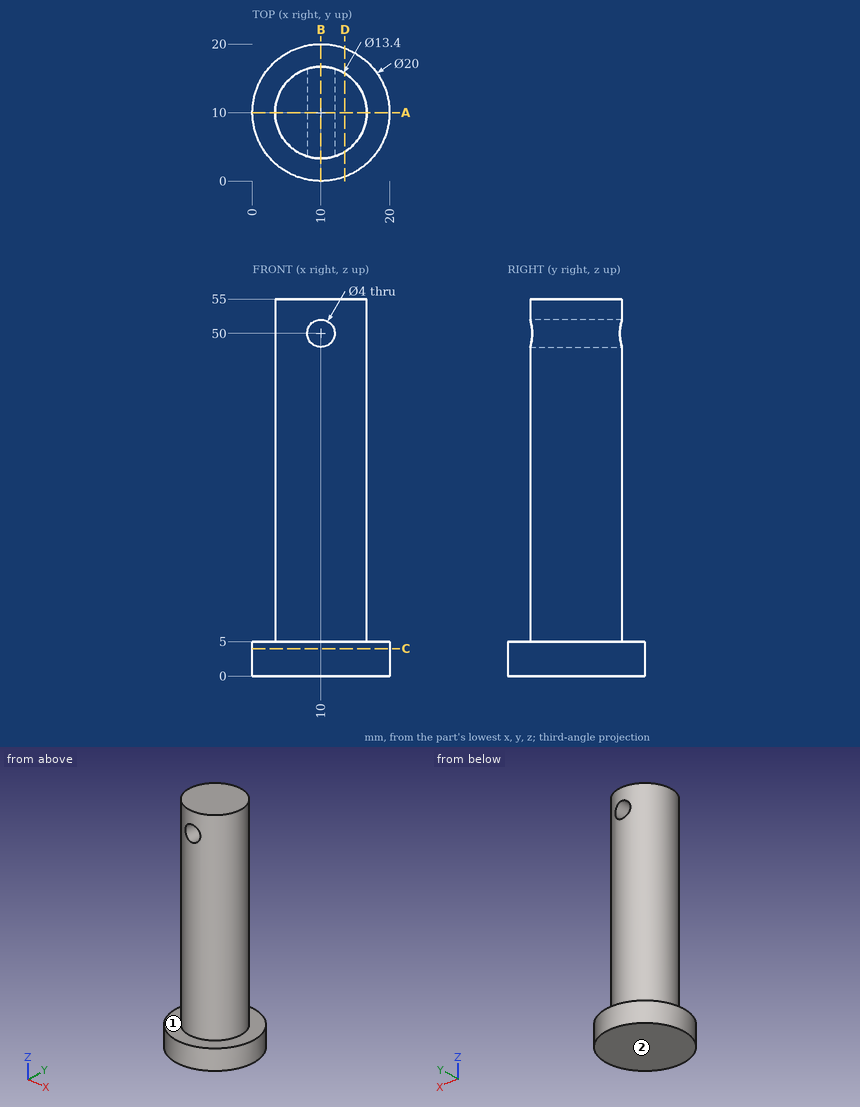
Verification items for this drawing (mm, ordinates from the low corner). A direction names the side the tool comes from. Round coordinates to 2 decimals unless told otherwise and drop trailing zeros. Loops run counter-clockwise (first coordinate to the right, second up) from the corner with the lowest first, then second, coordinate; pieces in that order, holes last. Notation, with made-up numbers: (62.25, 84.25) -> (92.25, 84.25) arc R24 ccw to (92.25, 121.25) -> close; hole circle Ø6 at (21.25, 68.5). An arc over 180 degrees is marked (long way). Write item = value, one per line. Start each with the question number.
1) Sectioned sample at C-C, the plane z = 4. Record the cut outline in (x, y), plus the area to 3 significant figures.
2) Sectioned sample at D-D, the plane x = 13.5. Record the cut outline in (y, z), plus the area to 3 significant figures.
3) Sectioned sample at A-A, the plane y = 10. Record the cut outline in (x, z), plus the area to 3 significant figures.
4) Set-up check for the marked faces 1 and 2: record each of +Z, -Z, +X, -X, +Y, -Y from which the full face is reachable in a straight line by a thin tool's end or side.
5) Gauge pin test, flat ends, axial feed: pin 1 Ø4 at (y, z) = (5.5, 13) entering from +X; pin 2 Ø8 at (y, z) = (10.5, 43.5) entering from +X; pin 3 Ø6.5 at (x, z) = (10, 50) entering from +Y. Record the tip position at first contact, or that the pin passes through.
6) Thickness scan on probe 1 along Z at (x, y) = (10, 12); probe 2 along X at (y, z) = (13, 50); probe 3 along X at (y, z) = (10.25, 22). Record the ranges inside material, lowest first.
7) Sectioned sample at B-B, the plane x = 10. Record the cut outline in (y, z), plus the area to 3 significant figures.
Results are:
q1.outline = circle Ø20 at (10, 10)
q1.area = 314 mm^2
q2.outline = (0.63, 0) -> (19.37, 0) -> (19.37, 5) -> (15.71, 5) -> (15.71, 55) -> (4.29, 55) -> (4.29, 5) -> (0.63, 5) -> close
q2.area = 665 mm^2
q3.outline = (0, 0) -> (20, 0) -> (20, 5) -> (16.7, 5) -> (16.7, 55) -> (3.3, 55) -> (3.3, 5) -> (0, 5) -> close; hole circle Ø4 at (10, 50)
q3.area = 757 mm^2
q4.face_1 = +Z
q4.face_2 = -Z, +X, -X, +Y, -Y
q5.pin_1 = 16.22
q5.pin_2 = 16.7
q5.pin_3 = 16.7
q6.probe_1 = 0 to 48, 52 to 55
q6.probe_2 = 4.01 to 8, 12 to 15.99
q6.probe_3 = 3.3 to 16.7
q7.outline = (0, 0) -> (20, 0) -> (20, 5) -> (16.7, 5) -> (16.7, 48) -> (3.3, 48) -> (3.3, 5) -> (0, 5) -> close; (3.3, 52) -> (16.7, 52) -> (16.7, 55) -> (3.3, 55) -> close
q7.area = 716 mm^2
